Autodesk Inventor part; units mm, degrees
ref_plane "YZ Plane" through (0, 0, 0) normal (1, 0, 0) x (0, 1, 0)
ref_plane "XZ Plane" through (0, 0, 0) normal (0, 1, 0) x (-1, 0, 0)
ref_plane "XY Plane" through (0, 0, 0) normal (0, 0, 1) x (1, 0, 0)
sketch "Esboço1" plane through (0, 0, 0) normal (0, 0, 1) x (1, 0, 0)
  line L0 (-14, 0) -> (-14, 5.25)
  line L1 (-14, 5.25) -> (-13.45, 5.25)
  line L2 (-13.45, 5.25) -> (-13.45, 6.85)
  line L3 (-13.45, 6.85) -> (-14, 6.85)
  line L4 (-14, 6.85) -> (-14, 30.15)
  line L5 (-14, 30.15) -> (-13.45, 30.15)
  line L6 (-13.45, 30.15) -> (-13.45, 31.75)
  line L7 (-13.45, 31.75) -> (-14, 31.75)
  line L8 (-14, 31.75) -> (-14, 37)
  line L9 (-14, 37) -> (-13, 37)
  line L10 (-14, 0) -> (-13, 0)
  line L11 (-13, 0) -> (0, 0) construction
  line L12 (0, 0) -> (0, 37) construction
  line L13 (0, 37) -> (-13, 37) construction
  line L14 (-13, 37) -> (-13, 0)
  dimension "d0" = 13
  dimension "d1" = 37
  dimension "d4" = 0.55
  dimension "d5" = 1.6
  dimension "d6" = 1.6
  dimension "d8" = 1
  dimension "d26" = 26.5
  dimension "d27" = 5.25
sketch "Esboço3" plane through (0, 0, 0) normal (0, 0, 1) x (1, 0, 0)
  line L0 (0, 37) -> (0, 0) construction
  line L1 (0, 37) -> (0, 35.5) construction
  line L2 (0, 0) -> (0, 1.5) construction
  line L3 (-8, 0) -> (-8, 37)
  line L4 (-8, 0) -> (-9.5, 0)
  line L5 (-9.5, 37) -> (-8, 37)
  line L6 (-9.5, 1.5) -> (-13, 1.5)
  line L7 (-13, 1.5) -> (-13, 35.5)
  line L8 (-13, 35.5) -> (-9.5, 35.5)
  line L9 (-9.5, 0) -> (-9.5, 1.5)
  line L10 (-9.5, 35.5) -> (-9.5, 37)
  dimension "d28" = 37
  dimension "d30" = 8
  dimension "d31" = 34
  dimension "d32" = 37
  dimension "d33" = 1.5
  dimension "d34" = 5
  dimension "d36" = 1.5
  dimension "d37" = 1.5
revolve "Revolução1" add sketch "Esboço3" angle 360 about axis through (0, 37, 0) along (0, -1, 0)
revolve "Revolução2" add sketch "Esboço1" angle 360 about axis through (0, 0, 0) along (0, 1, 0)
equation "\"d33\" = -0.5 * d31 + 0.5 * d32"
equation "\"d37\" = d36"
equation "\"d6\" = d5"
equation "\"d27\" = -0.5 * d26 + 0.5 * d1"
properties part number "rolamento_linear_lm16uu.iam"
CAD build for the part. Positions are in the model's coordinates, mm. A direction names the side the tool comes from. Round coordinates to 2 decimals unless told otherwise and drop trailing zeros. Loops run counter-clockwise (first coordinate to the right, second up) from the corner with the lowest first, then second, coordinate; pieces in that order, holes last. Notation, with made-up numbers: (81.5, -40) - (120.5, -40) arc R25 ccw to (120.5, -8) - close; hole circle Ø11 at (45, 61.5). An arc over 180 degrees is marked (long way). Put each result on its own line as item: value.
1. Slice it at A-A on y = 26. List the corners of the cut face in (x, z), and give its area (3 significant figures).
Geometry check:
outline: circle Ø28 at (0, 0); hole circle Ø16 at (0, 0)
area: 415 mm²
2. 3-axis set-ups, long thin cutter, end or side, ignore diameter. For faces 5 (the cylindrical face through (-4.38, 36.26, -8.43)), 6 (the cylindrical face through (-12.83, 6.06, 4.04)), 7 (the cylindrical face through (1.73, 18.76, -7.81)), 8 (the cylindrical face through (-4.38, 0.76, -8.43)), 9 (the flat face through (4.3, 0, 7)): which of +Z, -Z, +X, -X, +Y, -Y reach the whole face in a straight line?
Geometry check:
face 5: +Y
face 6: none
face 7: +Y, -Y
face 8: -Y
face 9: +Z, -Z, +X, -X, -Y
3. Pin check, flat tips, straight feed: P1, Ø5, axis at x = -3, z = 1.5, coming from the +Y side; P2, Ø1, axis at y = 14, z = -4, coming from the -X side; P3, Ø8, axis at y = 33.5, z = 11, coming from the -X side; P4, Ø14, axis at x = -2.5, z = -6, coming from the +Y side. Stop position of each tip, or through.
Geometry check:
P1: through
P2: x = -13.56
P3: x = -12.12
P4: y = 37
4. Two-plate mould, pull along Y, no slides. Class faces 1 (the cylindrical face through (10.316, 36.24, 7.91)), 2 (the flat face through (7.3, 6.85, 11.5)), 3 (the cylindrical face through (-12.83, 30.96, 4.04)), 4 (the flat face through (-9.3, 0, -9.3)): released by +Y, released by -Y, zero draft, split by the parting line, or undercut.
Geometry check:
face 1: zero draft
face 2: undercut
face 3: undercut
face 4: released by -Y
5. Wall check: line 1 (Z direction, x = 0, y = 36.35); line 2 (Z direction, x = 0, y = 21); line 3 (Z direction, x = -1.5, y = 27). Give the ranges that are in metal, low to high.
Geometry check:
line 1: -14 to -13, -9.5 to -8, 8 to 9.5, 13 to 14
line 2: -14 to -8, 8 to 14
line 3: -13.92 to -7.86, 7.86 to 13.92
